Here's how the part is built. I have some questions about the finished solid (model axes, mm). Face numbers are marked on the shaded views. A direction names the side the tool comes from. Give positions to 0.01 mm unless a question says otherwise; leave off trailing zeros. Loops run counter-clockwise (first coordinate to the right, second up) from the corner with the lowest first, then second, coordinate; pieces in that order, holes last. Notation, with made-up numbers: (54, 41.5) -> (58, 41.5) arc R23 ccw to (58, 68.5) -> close; hole circle Ø6 at (59, -35). An arc over 180 degrees is marked (long way). Answer in a Markdown table with one row per item. Add a question column.
Item 1: For P1, Ø5, axis at x = -10.85, y = -11.69, coming from the +Z side (3 decimals); P2, Ø10.5, axis at x = 1.5, y = -2.5, coming from the +Z side; P3, Ø1.8, axis at x = 11, y = 0.5, coming from the +Z side; P4, Ø2.5, axis at x = -10.85, y = 11.69, coming from the -Z side, each with a flat end and sliding along its axis, tell me the tip position at first contact or that it passes through.
Item 2: If we section it at D-D (y = 15): Write out the boundary of the cut face in (x, z) (3 decimals).
Item 3: Which directions (+Z, -Z, +X, -X, +Y, -Y) give clear straight access to the entire face, cutting with the end or side of a thin tool? Please do the marked faces 5 and 6.
Item 4: We'd pull the mould along X, two halves only. Please class the marked faces 1, 2, 3 and 4: released by +X, released by -X, zero draft, split by the parting line, or undercut.
Item 5: If we section it at A-A (z = 4.5): Give the number of separate pieces and of enclosed holes in the cut face, then the cut area to 3 significant figures.
Item 6: If I drill on line 1 (Y direction, x = -4.5, z = 6.5); line 2 (X direction, y = 0, z = 5); line 3 (Y direction, x = -11, z = 2.75), over which ranges is the centre line in solid material (lowest first)?
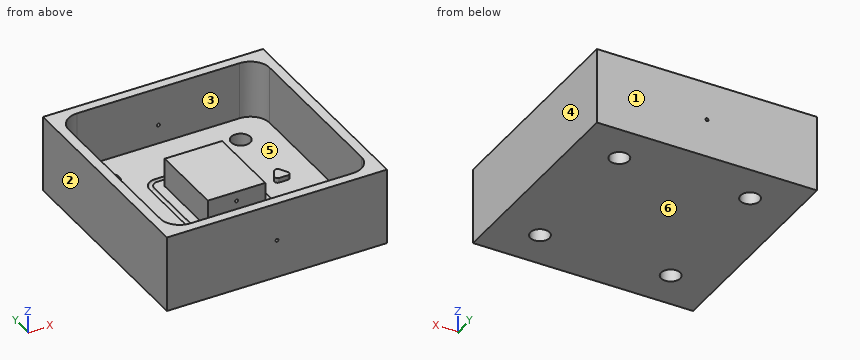
```python
from build123d import *

# Parameters (mm, degrees)
F0_W      = 36.5125
F0_H      = 36.5125
F1_DEPTH  = 12.7
F2_W      = 33.3375
F2_H      = 33.3375
F3_DEPTH  = 9.525
F4_W      = 9.525
F4_H      = 12.7
F5_DEPTH  = 4.7625
F7_D      = 0.508
F7_DEPTH  = 14.2875
F7_TIP    = 0.1526185972
F9_D      = 0.508
F9_DEPTH  = 14.2875
F9_TIP    = 0.1526185972
F10_R     = 3.175
F15_D     = 3.175
F17_DEPTH = 0.79375
F18_R     = 0.508


with BuildPart() as f1:
    # F0 (on Top) → F1 (new body)
    with BuildSketch(Plane.XY):
        Rectangle(F0_W, F0_H)
    extrude(amount=F1_DEPTH)

    # F2 (on face) → F3 (cut)
    with BuildSketch(Plane.XY.offset(12.7)):
        Rectangle(F2_W, F2_H)
    extrude(amount=-F3_DEPTH, mode=Mode.SUBTRACT)

    # F4 (on face) → F5 (join)
    with BuildSketch(Plane.XY.offset(3.175)):
        Rectangle(F4_W, F4_H)
    extrude(amount=F5_DEPTH)

    # F7
    with Locations(Plane.XZ.offset(18.25625)):
        with Locations((0, 6.35)):
            Hole(F7_D / 2, depth=F7_DEPTH)
            with Locations((0, 0, -(F7_DEPTH + F7_TIP / 2))):  # 118° drill point
                Cone(0, F7_D / 2, F7_TIP, mode=Mode.SUBTRACT)

    # F9
    with Locations(Plane(origin=(0, 18.25625, 0), x_dir=(-1, 0, 0), z_dir=(0, 1, 0))):
        with Locations((0, 6.35)):
            Hole(F9_D / 2, depth=F9_DEPTH)
            with Locations((0, 0, -(F9_DEPTH + F9_TIP / 2))):  # 118° drill point
                Cone(0, F9_D / 2, F9_TIP, mode=Mode.SUBTRACT)

    # F10
    f10_edges = [f1.edges().sort_by_distance(p)[0] for p in [
        (-16.66875, 16.66875, 7.9375),
        (-16.66875, -16.66875, 7.9375),
        (16.66875, -16.66875, 7.9375),
        (16.66875, 16.66875, 7.9375),
    ]]
    fillet(f10_edges, radius=F10_R)

    # F13: sweep along a path in F11
    with BuildLine(Plane.XY.offset(3.175)) as f13_path:
        Line((5.1181, -8.2931), (-5.1181, -8.2931))
        ThreePointArc((-5.1181, -8.2931), (-6.2406320151, -7.8281320151), (-6.7056, -6.7056))
        Line((-6.7056, -6.7056), (-6.7056, 0))
        Line((-6.7056, 0), (-6.7056, 6.7056))
        ThreePointArc((-6.7056, 6.7056), (-6.2406320151, 7.8281320151), (-5.1181, 8.2931))
        Line((-5.1181, 8.2931), (5.1181, 8.2931))
        ThreePointArc((5.1181, 8.2931), (6.2406320151, 7.8281320151), (6.7056, 6.7056))
        Line((6.7056, 6.7056), (6.7056, -6.7056))
        ThreePointArc((6.7056, -6.7056), (6.2406320151, -7.8281320151), (5.1181, -8.2931))
    # F12 (on Front) → F13 (sweep, cut)
    with BuildSketch(Plane.XZ):
        with BuildLine():
            Line((-6.3246, 3.175), (-7.0866, 3.175))
            ThreePointArc((-7.0866, 3.175), (-6.7056, 2.794), (-6.3246, 3.175))
        make_face()
    sweep(path=f13_path.line, mode=Mode.SUBTRACT)

    # F15 (through all)
    with Locations(Plane.XY.offset(3.175)):
        with Locations((10.8477650555, -11.6891054078), (10.8477650555, 11.6891054078), (-10.8477650555, 11.6891054078), (-10.8476863706, -11.689040258)):
            Hole(F15_D / 2)

    # F16 (on face) → F17 (join)
    with BuildSketch(Plane.XY.offset(3.175)):
        Polygon((9.2602650555, -0.9165435523), (12.4352650555, -0.9165435523), (10.8477650555, 1.8330871047), align=None)
    extrude(amount=F17_DEPTH)

    # F18
    f18_edges = [f1.edges().sort_by_distance(p)[0] for p in [
        (10.847765, 1.833087, 3.571875),
        (12.435265, -0.916544, 3.571875),
        (9.260265, -0.916544, 3.571875),
    ]]
    fillet(f18_edges, radius=F18_R)


solid = f1.part
```
Recorded:
| question | item | result |
|---|---|---|
| 1 | P1 | stops at z = 3.175 |
| 1 | P2 | stops at z = 7.94 |
| 1 | P3 | stops at z = 3.97 |
| 1 | P4 | passes through |
| 2 | outline | (-18.256, 0) -> (18.256, 0) -> (18.256, 12.7) -> (16.289, 12.7) -> (16.289, 3.175) -> (-16.289, 3.175) -> (-16.289, 12.7) -> (-18.256, 12.7) -> close |
| 3 | face 5 | +Z |
| 3 | face 6 | -Z, +X, -X, +Y, -Y |
| 4 | face 1 | zero draft |
| 4 | face 2 | released by -X |
| 4 | face 3 | undercut |
| 4 | face 4 | released by +X |
| 5 | separate pieces | 2 |
| 5 | enclosed holes | 1 |
| 5 | area | 351 mm^2 |
| 6 | line 1 | y = -18.26 to -16.67, -6.35 to 6.35, 16.67 to 18.26 |
| 6 | line 2 | x = -18.26 to -16.67, -4.76 to 4.76, 16.67 to 18.26 |
| 6 | line 3 | y = -18.26 to -13.27, -10.11 to 10.11, 13.27 to 18.26 |
